```python
from build123d import *

# Parameters (mm, degrees)
SKETCH_W        = 30
SKETCH_H        = 30
PAD_DEPTH       = 30
SKETCH001_W     = 25.5
SKETCH001_H     = 25.5
PAD001_DEPTH    = 50
CHAMFER_SIZE    = 2
SKETCH002_W     = 25.5
SKETCH002_H     = 25.5
PAD002_DEPTH    = 50
CHAMFER001_SIZE = 2
SKETCH003_W     = 25.5
SKETCH003_H     = 25.5
PAD003_DEPTH    = 50
CHAMFER002_SIZE = 2


with BuildPart() as part:
    # Sketch → Pad (new body)
    with BuildSketch(Plane.XY):
        Rectangle(SKETCH_W, SKETCH_H)
    extrude(amount=PAD_DEPTH)

    # Sketch001 (on Face2 of Pad) → Pad001 (join)
    with BuildSketch(Plane.XZ.offset(15)):
        with Locations((0, 15)):
            Rectangle(SKETCH001_W, SKETCH001_H)
    extrude(amount=PAD001_DEPTH)

    # Chamfer
    chamfer_edges = [part.edges().sort_by_distance(p)[0] for p in [
        (-12.75, -40, 27.75),
        (-12.75, -65, 15),
        (-12.75, -40, 2.25),
        (0, -65, 2.25),
        (12.75, -65, 15),
        (0, -65, 27.75),
        (12.75, -40, 27.75),
        (12.75, -40, 2.25),
    ]]
    chamfer(chamfer_edges, length=CHAMFER_SIZE)

    # Sketch002 (on Face10 of Chamfer) → Pad002 (join)
    with BuildSketch(Plane.YZ.offset(15)):
        with Locations((0, 15)):
            Rectangle(SKETCH002_W, SKETCH002_H)
    extrude(amount=PAD002_DEPTH)

    # Chamfer001
    chamfer001_edges = [part.edges().sort_by_distance(p)[0] for p in [
        (65, 12.75, 15),
        (40, 12.75, 27.75),
        (40, -12.75, 27.75),
        (65, 0, 27.75),
        (65, -12.75, 15),
        (65, 0, 2.25),
        (40, -12.75, 2.25),
        (40, 12.75, 2.25),
    ]]
    chamfer(chamfer001_edges, length=CHAMFER001_SIZE)

    # Sketch003 (on Face10 of Chamfer001) → Pad003 (join)
    with BuildSketch(Plane(origin=(0, 15, 0), x_dir=(-1, 0, 0), z_dir=(0, 1, 0))):
        with Locations((0, 15)):
            Rectangle(SKETCH003_W, SKETCH003_H)
    extrude(amount=PAD003_DEPTH)

    # Chamfer002
    chamfer002_edges = [part.edges().sort_by_distance(p)[0] for p in [
        (12.75, 40, 27.75),
        (-12.75, 40, 27.75),
        (0, 65, 27.75),
        (-12.75, 65, 15),
        (12.75, 65, 15),
        (12.75, 40, 2.25),
        (0, 65, 2.25),
        (-12.75, 40, 2.25),
    ]]
    chamfer(chamfer002_edges, length=CHAMFER002_SIZE)


solid = part.part
```
The model under review builds one solid part; all positions refer to its coordinate system, in mm. A direction names the side the tool comes from. Coordinates: 2 decimals unless noted, no trailing zeros. Write each loop counter-clockwise with the first axis right and the second up, starting at its lowest first coordinate (ties: lowest second). Pieces come first, ordered by that corner, then holes. Notation, with made-up numbers: (6.5, 14.5) - (22.5, 14.5) arc R25 cw to (22.5, 52.5) - close; hole circle Ø4 at (74, 30). An arc over 180 degrees is marked (long way). Answer in a Markdown table with one row per item. Add a question column.
Q1. To check wall thickness, follow line 1 along Z through (x, y) = (-10.5, -21); line 2 along X through (y, z) = (42, 13.75). State the ranges of each line that lie inside material, in increasing order. Write a range as from..to.
Q2. Consider section B-B on x = 3.5. Give the boundary of the cut face in (y, z).
Q3. Clearance check with flat-ended pins moving along their axes: pin 1 (10 mm diameter, centred on x = 52.5, z = 5, fed in from -Y); pin 2 (5 mm diameter, centred on y = -43, z = 5.5, fed in from -X); pin 3 (23.5 mm diameter, centred on x = -1.5, y = -40, fed in from +Z). State where each tip first meets the part, or that it passes through.
Q4. For faces 1 (the face through (0, 39, 2.25)), 2 (the face through (-14, -15, 15)), 3 (the face through (12.75, -39, 15)), 4 (the face through (39, 0, 27.75)), list the 3-axis set-ups (+Z, -Z, +X, -X, +Y, -Y) from which the entire face can be reached by the end or side of a thin tool; tool diameter is ignored.
Q5. Consider section A-A on z = 18.5. Give the boundary of the cut face in (x, y), then the cut area to 3 significant figures.
Q6. Consider section C-C on y = -46.5. Give the boundary of the cut face in (x, z).
Answers below:
| question | item | result |
|---|---|---|
| 1 | line 1 | 2.25..27.75 |
| 1 | line 2 | -12.75..12.75 |
| 2 | outline | (-65, 4.25) - (-63, 2.25) - (-15, 2.25) - (-15, 0) - (15, 0) - (15, 2.25) - (63, 2.25) - (65, 4.25) - (65, 25.75) - (63, 27.75) - (15, 27.75) - (15, 30) - (-15, 30) - (-15, 27.75) - (-63, 27.75) - (-65, 25.75) - close |
| 3 | pin 1 | y = -12.75 |
| 3 | pin 2 | x = -12.75 |
| 3 | pin 3 | z = 27.75 |
| 4 | face 1 | -Z, +X, -X, +Y |
| 4 | face 2 | -Y |
| 4 | face 3 | +Z, -Z, +X, -Y |
| 4 | face 4 | +Z, +X, +Y, -Y |
| 5 | outline | (-15, -15) - (-12.75, -15) - (-12.75, -63) - (-10.75, -65) - (10.75, -65) - (12.75, -63) - (12.75, -15) - (15, -15) - (15, -12.75) - (63, -12.75) - (65, -10.75) - (65, 10.75) - (63, 12.75) - (15, 12.75) - (15, 15) - (12.75, 15) - (12.75, 63) - (10.75, 65) - (-10.75, 65) - (-12.75, 63) - (-12.75, 15) - (-15, 15) - close |
| 5 | area | 4,710 mm² |
| 6 | outline | (-12.75, 4.25) - (-10.75, 2.25) - (10.75, 2.25) - (12.75, 4.25) - (12.75, 25.75) - (10.75, 27.75) - (-10.75, 27.75) - (-12.75, 25.75) - close |
